```python
from build123d import *

# Parameters (mm, degrees)
F1_DEPTH = 63.5
F2_DEPTH = 25.4
F3_DEPTH = 7.9375
F5_R     = 6.35


with BuildPart() as f1:
    # F0 (on Front) → F1 (new body, symmetric)
    with BuildSketch(Plane.XZ):
        Polygon((-41.275, -9.525), (41.275, -9.525), (41.275, 9.525), (22.225, 9.525), (-41.275, 9.525), align=None)
    extrude(amount=F1_DEPTH, both=True)

    # F0 (on Front) → F2 (join, symmetric)
    with BuildSketch(Plane.XZ):
        with BuildLine():
            Line((22.225, 9.525), (41.275, 9.525))
            Line((41.275, 9.525), (41.275, 22.81095))
            ThreePointArc((41.275, 22.81095), (46.796103, 36.644574), (60.325, 42.8752))
            Line((60.325, 42.8752), (60.325, 61.9252))
            Line((60.325, 61.9252), (59.912667, 61.9252))
            ThreePointArc((59.912667, 61.9252), (33.179972, 49.969212), (22.225, 22.81095))
            Line((22.225, 22.81095), (22.225, 9.525))
        make_face()
    extrude(amount=F2_DEPTH, both=True)

    # F0 (on Front) → F3 (join, symmetric)
    with BuildSketch(Plane.XZ):
        with BuildLine():
            add(Edge.make_bspline(
                [(-41.275, 9.525), (-25.498318, 48.070595), (22.572279, 65.208808), (59.912667, 61.9252)],
                knots=[0, 0, 0, 0, 113.950537, 113.950537, 113.950537, 113.950537], degree=3))
            Line((-41.275, 9.525), (22.225, 9.525))
            Line((22.225, 9.525), (22.225, 22.81095))
            ThreePointArc((22.225, 22.81095), (33.179972, 49.969212), (59.912667, 61.9252))
        make_face()
    extrude(amount=F3_DEPTH, both=True)

    # F0 (on Front) → F4 (revolve)
    with BuildSketch(Plane.XZ):
        Polygon((84.855057, 42.8752), (60.325, 42.8752), (60.325, 38.1), (111.125, 38.1), (111.125, 66.675), (60.325, 66.675), (60.325, 61.9252), (84.855057, 61.9252), align=None)
    revolve(axis=Axis((60.325, 0, 52.3875), (0, 0, 1)))

    # F5
    f5_edges = [f1.edges().sort_by_distance(p)[0] for p in [
        (-41.275, -63.5, 0),
        (41.275, -63.5, 0),
        (-41.275, 63.5, 0),
        (41.275, 63.5, 0),
    ]]
    fillet(f5_edges, radius=F5_R)


solid = f1.part
```
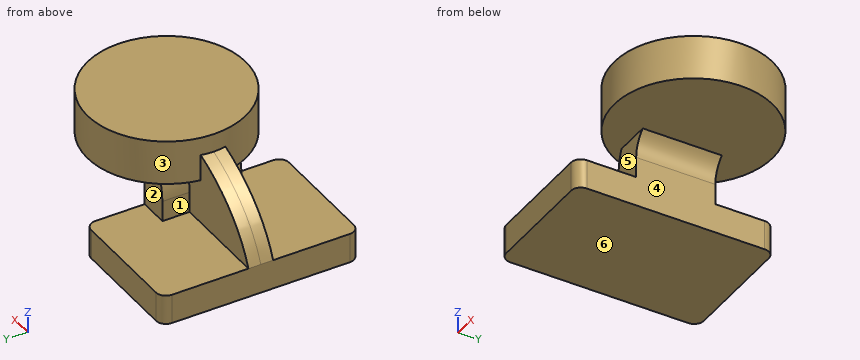
The model under review builds one solid part; all positions refer to its coordinate system, in mm. Face numbers are marked on the shaded views. A direction names the side the tool comes from. Round coordinates to 2 decimals unless told otherwise and drop trailing zeros. Write each loop counter-clockwise with the first axis right and the second up, starting at its lowest first coordinate (ties: lowest second). Pieces come first, ordered by that corner, then holes. Notation, with made-up numbers: M 14.25,-8.75 L 68.25,-8.75 A11 ccw 68.25,12.25 Z; hole C 50.5,-15 d6. An arc over 180 degrees is marked long. Use CSV: the item, a comma, the result in double quotes. Start each with the question number.
(1) For line 1 along Z through (x, y) = (40, 25.5) (3 decimals); line 2 along Z through (x, y) = (100.5, -28.5) (3 decimals); line 3 along Y through (x, z) = (36.5, 31.5), list the stretches that pass through material, from the lowest coordinate up.
(2) The part is to be moulded in two halves that separate along Z. For the marked faces 4, 5 and 6, say which applies: +Z half, -Z half, draft (parallel to the pull), parting line (faces both ways), or undercut.
(3) We need section D-D, the plane x = 101.5. State the section outline as (y, z) points (3 decimals), then the cut area to 3 significant figures.
(4) We need section C-C, the plane x = 81. State the section outline as (y, z) points (3 decimals), then the cut area to 3 significant figures.
(5) We need section A-A, the plane y = 13. State the section outline as (x, z) points (1 decimal).
(6) Clearance check with flat-ended pins moving along their axes: P1, Ø5, axis at x = 9, y = -8, coming from the +Z side (3 decimals); P2, Ø8, axis at x = 30.5, z = 28, coming from the +Y side; P3, Ø5, axis at x = 5.5, z = 45, coming from the +Y side; P4, Ø23, axis at x = 5.5, z = 32, coming from the +Y side. State where each tip first meets the part, or that it passes through.
(7) Tool access review of the marked faces 1, 2 and 3: name each direction out of +Z, -Z, +X, -X, +Y, -Y from which nothing blocks a thin tool from reaching the whole face with its end or side.
(8) We need section B-B, the plane z = 5. State the section outline as (x, y) points (3 decimals), then the cut area to 3 significant figures.
Findings:
1,line 1,"-9.525 to 9.525, 38.1 to 66.675"
1,line 2,"38.1 to 66.675"
1,line 3,"-25.4 to 25.4"
2,face 4,"draft"
2,face 5,"undercut"
2,face 6,"-Z half"
3,outline,"M -29.753,38.1 L 29.753,38.1 L 29.753,66.675 L -29.753,66.675 Z"
3,area,"1,700 mm^2"
4,outline,"M -46.402,38.1 L 46.402,38.1 L 46.402,66.675 L -46.402,66.675 Z; hole M -13.201,42.875 L 13.201,42.875 L 13.201,61.925 L -13.201,61.925 Z"
4,area,"2,150 mm^2"
5,outline,"M -41.3,-9.5 L 41.3,-9.5 L 41.3,22.8 A20.1 cw 48.3,38.1 L 109.4,38.1 L 109.4,66.7 L 11.2,66.7 L 11.2,38.1 L 25.3,38.1 A39.1 ccw 22.2,22.8 L 22.2,9.5 L -41.3,9.5 Z; hole M 39.5,55.3 A39.1 cw 59.9,61.9 L 39.5,61.9 Z; hole M 60.3,42.9 L 81.1,42.9 L 81.1,61.9 L 60.3,61.9 Z"
6,P1,"z = 66.675"
6,P2,"y = 25.4"
6,P3,"y = 7.94"
6,P4,"y = 23.43"
7,face 1,"-X, +Y"
7,face 2,"+X, -X, +Y"
7,face 3,"+Z"
8,outline,"M -41.275,-57.15 A6.35 ccw -34.925,-63.5 L 34.925,-63.5 A6.35 ccw 41.275,-57.15 L 41.275,57.15 A6.35 ccw 34.925,63.5 L -34.925,63.5 A6.35 ccw -41.275,57.15 Z"
8,area,"10,400 mm^2"
